Read the model definition and answer for the solid it produces. Units are mm, in the model's axes. A direction names the side the tool comes from. Give positions to 0.01 mm unless a question says otherwise; leave off trailing zeros. Loops run counter-clockwise (first coordinate to the right, second up) from the corner with the lowest first, then second, coordinate; pieces in that order, holes last.
(1) Which of the six approach directions +Z, -Z, +X, -X, +Y, -Y give full straight-line access (tool end or side, diameter ignored) to faces 1 (the face through (-4, 8, 4)), 2 (the face through (-46.5, 7, 4.1)), 3 (the face through (-133.584, 6.766, 4.056))?
(2) Find section B-B, the plane y = 12.75. Write down the section's boundary in (x, z).
(3) Each of these flat-tipped pins is pushed along its axis until it touches: P1, Ø2, axis at y = 7, z = 5.5, coming from the -X side; P2, Ø2, axis at y = 23.5, z = 2.5, coming from the -X side. Where does it stop, or does it pass through?
(4) Determine the mould class of faces 4 (the face through (-58, 45, 4)), 5 (the face through (-60, 0, 4)), 6 (the face through (-43, 8.5, 4)) for opening direction Y: pulls with the +Y half, pulls with the -Y half, needs draft (parallel to the pull), parting line crosses it, or undercut.
(5) Find section D-D, the plane y = 29. Write down the section's boundary in (x, z).
(6) Straight lines are drawn through the part: probe 1 along Y at (x, z) = (-117.5, 3); probe 2 along Y at (x, z) = (-18, 4.25); probe 3 along X at (y, z) = (23, 0.75). For each, find the intervals that lie inside material, in ascending order.
(7) Find section C-C, the plane z = 4.5. State how many separate pieces and enclosed holes the cut face has, then the cut area to 3 significant figures.
(8) Find section A-A, the plane x = -18. Write down the section's boundary in (y, z), then the cut area to 3 significant figures.
```python
from build123d import *

# Parameters (mm, degrees)
BOSS_EXTRUDE1_DEPTH = 8
SKETCH5_R           = 12
CUT_EXTRUDE4_DEPTH  = 8
FILLET6_R           = 22.5
SKETCH6_R           = 1.5
CUT_EXTRUDE5_DEPTH  = 8
CUT_EXTRUDE6_DEPTH  = 10
SKETCH11_R          = 1.5
CUT_EXTRUDE7_DEPTH  = 8


with BuildPart() as part:
    # Sketch1 → Boss-Extrude1 (new body)
    with BuildSketch(Plane.XY):
        Polygon((-8, 37), (0, 37), (0, 45), (-140, 45), (-140, 22.5), (-140, 0), (0, 0), (0, 8), (-8, 8), align=None)
    extrude(amount=BOSS_EXTRUDE1_DEPTH)

    # Sketch5 → Cut-Extrude4 (cut)
    with BuildSketch(Plane.XY.offset(8)):
        with Locations((-117.5, 22.5)):
            Circle(SKETCH5_R)
    extrude(amount=-CUT_EXTRUDE4_DEPTH, mode=Mode.SUBTRACT)

    # Fillet6
    fillet6_edges = [part.edges().sort_by_distance(p)[0] for p in [
        (-140, 45, 4),
        (-140, 0, 4),
    ]]
    fillet(fillet6_edges, radius=FILLET6_R - 0.0001)  # a hair under: the kernel refuses the full size

    # Sketch6 → Cut-Extrude5 (cut)
    with BuildSketch(Plane.XY.offset(8)):
        with Locations((-18, 12.75)):
            Circle(SKETCH6_R)
        with Locations((-18, 32.25)):
            Circle(SKETCH6_R)
        with Locations((-30.5, 32.25)):
            Circle(SKETCH6_R)
        with Locations((-30.5, 12.75)):
            Circle(SKETCH6_R)
    extrude(amount=-CUT_EXTRUDE5_DEPTH, mode=Mode.SUBTRACT)

    # Sketch7 → Cut-Extrude6 (cut)
    with BuildSketch(Plane.XY.offset(8)):
        with BuildLine():
            Line((-76, 39.5), (-71, 39.5))
            ThreePointArc((-71, 39.5), (-69.5, 38), (-71, 36.5))
            Line((-71, 36.5), (-76, 36.5))
            ThreePointArc((-76, 36.5), (-77.5, 38), (-76, 39.5))
        make_face()
        with BuildLine():
            Line((-45, 39.5), (-40, 39.5))
            ThreePointArc((-40, 39.5), (-38.5, 38), (-40, 36.5))
            Line((-40, 36.5), (-45, 36.5))
            ThreePointArc((-45, 36.5), (-46.5, 38), (-45, 39.5))
        make_face()
        with BuildLine():
            Line((-45, 8.5), (-40, 8.5))
            ThreePointArc((-40, 8.5), (-38.5, 7), (-40, 5.5))
            Line((-40, 5.5), (-45, 5.5))
            ThreePointArc((-45, 5.5), (-46.5, 7), (-45, 8.5))
        make_face()
        with BuildLine():
            Line((-76, 8.5), (-71, 8.5))
            ThreePointArc((-71, 8.5), (-69.5, 7), (-71, 5.5))
            Line((-71, 5.5), (-76, 5.5))
            ThreePointArc((-76, 5.5), (-77.5, 7), (-76, 8.5))
        make_face()
    extrude(amount=-CUT_EXTRUDE6_DEPTH, mode=Mode.SUBTRACT)

    # Sketch11 → Cut-Extrude7 (cut)
    with BuildSketch(Plane.XY.offset(8)):
        with Locations((-134.75, 22.5)):
            Circle(SKETCH11_R)
        with Locations((-117.5, 5.25)):
            Circle(SKETCH11_R)
        with Locations((-117.5, 39.75)):
            Circle(SKETCH11_R)
    extrude(amount=-CUT_EXTRUDE7_DEPTH, mode=Mode.SUBTRACT)


solid = part.part
```
Entries:
1. face 1: +Z, -Z, +X
1. face 2: +Z, -Z
1. face 3: +Z, -Z, -X, -Y
2. outline: (-137.78, 0) - (-124.5, 0) - (-124.5, 8) - (-137.78, 8) - close; (-110.5, 0) - (-32, 0) - (-32, 8) - (-110.5, 8) - close; (-29, 0) - (-19.5, 0) - (-19.5, 8) - (-29, 8) - close; (-16.5, 0) - (-8, 0) - (-8, 8) - (-16.5, 8) - close
3. P1: stops at x = -134.7
3. P2: stops at x = -140
4. face 4: pulls with the +Y half
4. face 5: pulls with the -Y half
4. face 6: undercut
5. outline: (-139.04, 0) - (-127.59, 0) - (-127.59, 8) - (-139.04, 8) - close; (-107.41, 0) - (-8, 0) - (-8, 8) - (-107.41, 8) - close
6. probe 1: y = 0 to 3.75, 6.75 to 10.5, 34.5 to 38.25, 41.25 to 45
6. probe 2: y = 0 to 11.25, 14.25 to 30.75, 33.75 to 45
6. probe 3: x = -139.99 to -136.16, -133.34 to -129.49, -105.51 to -8
7. separate pieces: 1
7. enclosed holes: 12
7. area: 5,260 mm2
8. outline: (0, 0) - (11.25, 0) - (11.25, 8) - (0, 8) - close; (14.25, 0) - (30.75, 0) - (30.75, 8) - (14.25, 8) - close; (33.75, 0) - (45, 0) - (45, 8) - (33.75, 8) - close
8. area: 312 mm2
